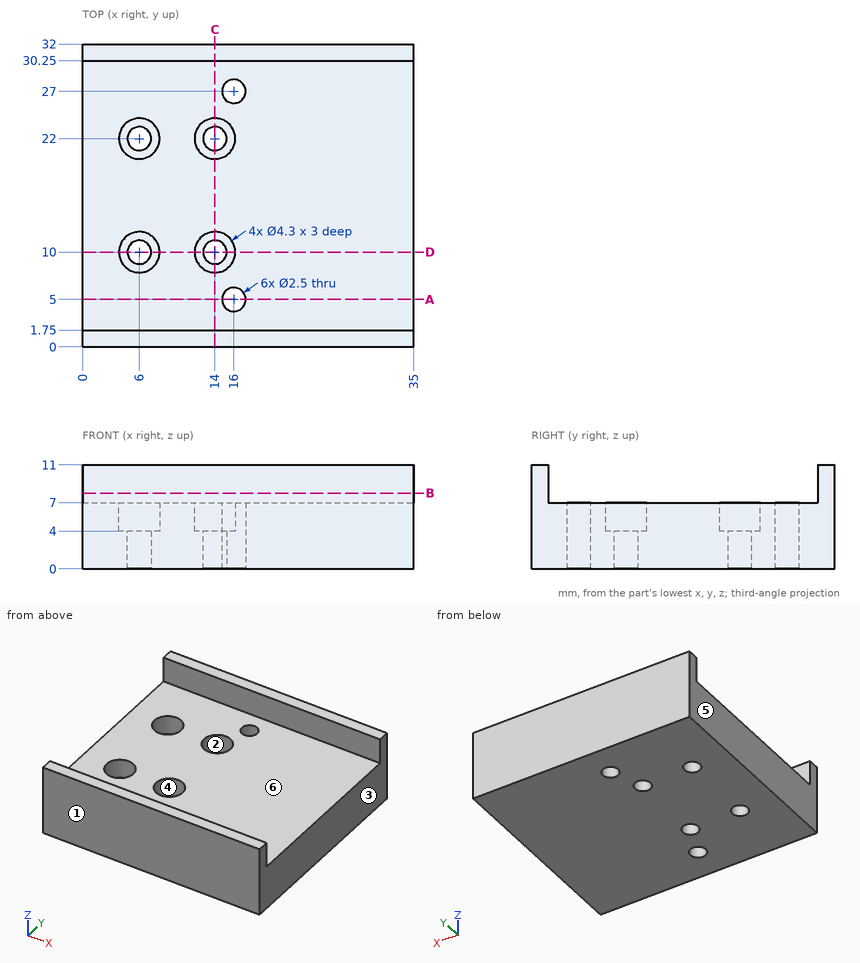
Can you work these out from the drawing? Everything is in mm from the part's minimum corner. A direction names the side the tool comes from. Coordinates: 2 decimals unless noted, no trailing zeros. Write each loop counter-clockwise with the first axis right and the second up, starting at its lowest first coordinate (ties: lowest second). Pieces come first, ordered by that corner, then holes. Notation, with made-up numbers: (-31, 39.5) -> (-20, 39.5) arc R8 cw to (-20, 44.5) -> close; hole circle Ø4 at (86, 56.25). An arc over 180 degrees is marked (long way). Write item = value, one per line.
(1) Imagine slicing it at B-B (z = 8). Please give me the cut outline in (x, y), and give its area (4 significant figures).
Verdict:
outline = (0, 0) -> (35, 0) -> (35, 1.75) -> (0, 1.75) -> close; (0, 30.25) -> (35, 30.25) -> (35, 32) -> (0, 32) -> close
area = 122.5 mm^2
(2) If I drill on probe 1 along Y at (x, z) = (6, 6.15); probe 2 along Y at (x, z) = (16, 1.5); probe 3 along Y at (x, z) = (15, 8.5), over which ranges is the centre line in solid material (lowest first)?
Verdict:
probe_1 = 0 to 7.85, 12.15 to 19.85, 24.15 to 32
probe_2 = 0 to 3.75, 6.25 to 25.75, 28.25 to 32
probe_3 = 0 to 1.75, 30.25 to 32
(3) For pin 1 (5.5 mm diameter, centred on x = 14, y = 22, fed in from +Z); pin 2 (5.5 mm diameter, centred on x = 6, y = 22, fed in from -Z); pin 3 (1.3 mm diameter, centred on x = 13, y = 11, fed in from +Z), each with a flat end and sliding along its axis, tell me the tip position at first contact or that it passes through.
Verdict:
pin_1 = 7
pin_2 = 0
pin_3 = 4
(4) Imagine slicing it at A-A (y = 5). Please give me the cut outline in (x, z), and give its area (4 significant figures).
Verdict:
outline = (0, 0) -> (14.75, 0) -> (14.75, 7) -> (0, 7) -> close; (17.25, 0) -> (35, 0) -> (35, 7) -> (17.25, 7) -> close
area = 227.5 mm^2
(5) Imagine slicing it at C-C (x = 14). Please give me the cut outline in (y, z), and give its area (3 significant figures).
Verdict:
outline = (0, 0) -> (8.75, 0) -> (8.75, 4) -> (7.85, 4) -> (7.85, 7) -> (1.75, 7) -> (1.75, 11) -> (0, 11) -> close; (11.25, 0) -> (20.75, 0) -> (20.75, 4) -> (19.85, 4) -> (19.85, 7) -> (12.15, 7) -> (12.15, 4) -> (11.25, 4) -> close; (23.25, 0) -> (32, 0) -> (32, 11) -> (30.25, 11) -> (30.25, 7) -> (24.15, 7) -> (24.15, 4) -> (23.25, 4) -> close
area = 192 mm^2
(6) On a 3-axis mill with a long thin cutter (end or side, diameter ignored), from which of +Z, -Z, +X, -X, +Y, -Y can I reach the whole of each face in a straight line? I mean the marked faces 4, 5 and 6. Say none if no direction works.
Verdict:
face_4 = +Z
face_5 = +Z, -Z, -X, +Y, -Y
face_6 = +Z, +X, -X
(7) Thinking about a two-plate mould opening in X: for the marked faces 1, 2 and 3, which applies, +X half, -X half, draft (parallel to the pull), parting line (faces both ways), or undercut?
Verdict:
face_1 = draft
face_2 = undercut
face_3 = +X half
(8) Imagine slicing it at D-D (y = 10). Please give me the cut outline in (x, z), and give its area (3 significant figures).
Verdict:
outline = (0, 0) -> (4.75, 0) -> (4.75, 4) -> (3.85, 4) -> (3.85, 7) -> (0, 7) -> close; (7.25, 0) -> (12.75, 0) -> (12.75, 4) -> (11.85, 4) -> (11.85, 7) -> (8.15, 7) -> (8.15, 4) -> (7.25, 4) -> close; (15.25, 0) -> (35, 0) -> (35, 7) -> (16.15, 7) -> (16.15, 4) -> (15.25, 4) -> close
area = 199 mm^2
